Autodesk Inventor part; units mm, degrees
ref_plane "YZ Plane" through (0, 0, 0) normal (1, 0, 0) x (0, 1, 0)
ref_plane "XZ Plane" through (0, 0, 0) normal (0, 1, 0) x (-1, 0, 0)
ref_plane "XY Plane" through (0, 0, 0) normal (0, 0, 1) x (1, 0, 0)
sketch "Sketch1" plane through (0, 0, 0) normal (0, 0, 1) x (1, 0, 0)
  line L0 (0, 0) -> (330.2, 0)
  line L1 (330.2, 0) -> (330.2, 95.25)
  line L2 (330.2, 95.25) -> (0, 95.25)
  line L3 (0, 95.25) -> (0, 0)
  dimension "d0" = 95.25
  dimension "d1" = 330.2
extrude "Extrusion1" add sketch "Sketch1" along normal blind 390.525
sketch "Sketch2" plane through (0, 95.25, 0) normal (0, 1, 0) x (1, 0, 0)
  line L0 (330.2, 0) -> (330.2, -390.525)
  line L1 (0, 0) -> (0, -390.525)
  line L2 (172.1995, -415.925) -> (330.2, -415.925)
  line L3 (330.2, -415.925) -> (330.2, -390.525)
  line L4 (152.4, -422.275) -> (0, -422.275)
  line L5 (0, -422.275) -> (0, -390.525)
  line L6 (159.1248, -420.6875) -> (165.4748, -417.5125)
  arc A0 (172.1995, -415.925) -> (165.4748, -417.5125) centre (172.1995, -430.962) ccw
  arc A1 (152.4, -422.275) -> (159.1248, -420.6875) centre (152.4, -407.238) ccw
  line L7 (330.2, -390.525) -> (0, -390.525)
  dimension "d4" = 25.4
  dimension "d6" = 152.4
  dimension "d7" = 6.35
  dimension "d8" = 3.175
  dimension "d9" = 31.75
  dimension "d10" = 158.0005
extrude "Extrusion2" add sketch "Sketch2" against normal blind 37.084
sketch "Sketch3" plane through (0, 0, 0) normal (0, -1, 0) x (1, 0, 0)
  line L0 (330.2, 0) -> (330.2, 390.525)
  line L1 (0, 390.525) -> (330.2, 390.525)
  line L2 (330.2, 390.525) -> (330.2, 419.1)
  line L3 (330.2, 419.1) -> (0, 419.1)
  line L4 (0, 419.1) -> (0, 390.525)
  dimension "d13" = 28.575
extrude "Extrusion3" add sketch "Sketch3" against normal blind 46.99
fillet "Fillet1" radius 4.318 4 edges at (330.2, 76.708, 415.925) (0, 76.708, 422.275) (0, 23.495, 419.1) (330.2, 23.495, 419.1)
sketch "Sketch4" plane through (0, 0, 0) normal (0, 0, -1) x (-1, 0, 0)
  line L0 (0, 95.25) -> (0, 0)
  line L1 (-330.2, 95.25) -> (0, 95.25)
  line L2 (-152.0825, 88.9) -> (-68.2625, 88.9)
  line L3 (-68.2625, 88.9) -> (-68.2625, 85.09)
  line L4 (-68.2625, 85.09) -> (-152.0825, 85.09)
  line L5 (-152.0825, 85.09) -> (-152.0825, 88.9)
  dimension "d17" = 68.2625
  dimension "d18" = 6.35
  dimension "d19" = 83.82
  dimension "d20" = 3.81
extrude "Extrusion4" add sketch "Sketch4" along normal blind 15.875
properties part number "PC"
Source: CAD feature listing. Evaluate the final solid. Frame: model axes, mm. A direction names the side the tool comes from. Give positions to 0.01 mm unless a question says otherwise; leave off trailing zeros. Write each loop counter-clockwise with the first axis right and the second up, starting at its lowest first coordinate (ties: lowest second). Pieces come first, ordered by that corner, then holes. Notation, with made-up numbers: M 46.25,66.5 L 94.25,66.5 A20 ccw 94.25,101.5 Z; hole C 4.25,70.5 d11. An arc over 180 degrees is marked long. Return JSON: item names as keys, results as strings. Group by question number.
1) Draft query along Y for faces 1 (the face through (248, 77, 415.925)), 2 (the face through (167, 95.25, 208)), 3 (the face through (163, 58.166, 406)). Return one class per face: released by +Y, released by -Y, zero draft, split by the parting line, or undercut.
2) Set-up query: faces 4 (the face through (163, 53, 390.525)), 5 (the face through (111, 88.9, -8)), 6 (the face through (330.2, 47, 204)), 7 (the face through (167, 23, 419.1)), 8 (the face through (110, 85.09, -8)). Return all of +Z, -Z, +X, -X, +Y, -Y with unobstructed straight access to the full face (end or side cutting, diameter ignored); none if empty.
3) Cut plane D-D, the plane x = 26.5. Output: boundary loops of the cut face in (y, z) (3 decimals), then the cut area to 3 significant figures.
4) First-contact query: pin 1 Ø4 at (x, y) = (118.5, 17) entering from +Z; pin 2 Ø3.5 at (x, y) = (222, 51.5) entering from +Z (3 decimals); pin 3 Ø6 at (x, y) = (128, 34.5) entering from -Z. Flat tips, straight axial feed; report the tip coordinate or a pass-through.
5) Cut plane C-C, the plane y = 25. Output: boundary loops of the cut face in (x, z), then the cut area to 3 significant figures.
6) Cut plane A-A, the plane y = 67.5. Output: boundary loops of the cut face in (x, z) (1 decimal).
7) Ray query, L1, parallel to Z at x = 30, y = 39.5; L2, parallel to Z at x = 212, y = 51 (3 decimals). Return the intervals inside material, ascending.
8) Cut plane B-B, the plane x = 193. Output: boundary loops of the cut face in (y, z) (3 decimals), then the cut area to 3 significant figures.
Data:
{
 "1": {"face 1": "zero draft", "face 2": "released by +Y", "face 3": "undercut"},
 "2": {"face 4": "+Z, +X, -X", "face 5": "-Z, +X, -X, +Y", "face 6": "+Z, -Z, +X, +Y, -Y", "face 7": "+Z, +X, -X, -Y", "face 8": "-Z, +X, -X, -Y"},
 "3": {"outline": "M 0,0 L 95.25,0 L 95.25,422.275 L 58.166,422.275 L 58.166,390.525 L 46.99,390.525 L 46.99,419.1 L 0,419.1 Z", "area": "39,700 mm²"},
 "4": {"pin 1": "stops at z = 419.1", "pin 2": "stops at z = 390.525", "pin 3": "stops at z = 0"},
 "5": {"outline": "M 0,0 L 330.2,0 L 330.2,414.78 A4.32 ccw 325.88,419.1 L 4.32,419.1 A4.32 ccw 0,414.78 Z", "area": "138,000 mm²"},
 "6": {"outline": "M 0,0 L 330.2,0 L 330.2,411.6 A4.3 ccw 325.9,415.9 L 172.2,415.9 A15 cw 165.5,417.5 L 159.1,420.7 A15 ccw 152.4,422.3 L 4.3,422.3 A4.3 ccw 0,418 Z"},
 "7": {"L1": "z = 0 to 419.1", "L2": "z = 0 to 390.525"},
 "8": {"outline": "M 0,0 L 95.25,0 L 95.25,415.925 L 58.166,415.925 L 58.166,390.525 L 46.99,390.525 L 46.99,419.1 L 0,419.1 Z", "area": "39,500 mm²"}
}
